from build123d import *

# Parameters (mm, degrees)
SKETCH1_R           = 1.6
BOSS_EXTRUDE1_DEPTH = 8
CHAMFER1_SIZE       = 1
SKETCH2_R           = 1.6
BOSS_EXTRUDE3_DEPTH = 8
FILLET1_R           = 10
CHAMFER2_SIZE       = 1


with BuildPart() as part:
    # Sketch1 → Boss-Extrude1 (new body)
    with BuildSketch(Plane.XY):
        with BuildLine():
            Line((-0.5, 3), (30.5, 3))
            ThreePointArc((30.5, 3), (32.267766953, 2.267766953), (33, 0.5))
            Line((33, 0.5), (33, -0.5))
            ThreePointArc((33, -0.5), (32.267766953, -2.267766953), (30.5, -3))
            Line((30.5, -3), (-0.5, -3))
            ThreePointArc((-0.5, -3), (-2.267766953, -2.267766953), (-3, -0.5))
            Line((-3, -0.5), (-3, 0.5))
            ThreePointArc((-3, 0.5), (-2.267766953, 2.267766953), (-0.5, 3))
        make_face()
        Circle(SKETCH1_R, mode=Mode.SUBTRACT)
        with Locations((7.5, 0)):
            Circle(SKETCH1_R, mode=Mode.SUBTRACT)
        with Locations((15, 0)):
            Circle(SKETCH1_R, mode=Mode.SUBTRACT)
        with Locations((22.5, 0)):
            Circle(SKETCH1_R, mode=Mode.SUBTRACT)
        with Locations((30, 0)):
            Circle(SKETCH1_R, mode=Mode.SUBTRACT)
    extrude(amount=BOSS_EXTRUDE1_DEPTH)

    # Chamfer1
    chamfer1_edges = [part.edges().sort_by_distance(p)[0] for p in [
        (-1.6, 0, 0),
        (-1.6, 0, 8),
        (5.9, 0, 0),
        (5.9, 0, 8),
        (13.4, 0, 0),
        (13.4, 0, 8),
        (20.9, 0, 0),
        (20.9, 0, 8),
        (28.4, 0, 0),
        (28.4, 0, 8),
    ]]
    chamfer(chamfer1_edges, length=CHAMFER1_SIZE)

    # Sketch2 → Boss-Extrude3 (add)
    with BuildSketch(Plane.XY.offset(8)):
        with BuildLine():
            ThreePointArc((-3, 0.5), (-2.809698831, 1.456708581), (-2.267766953, 2.267766953))
            Line((-2.267766953, 2.267766953), (-18.529200529, -13.993666623))
            ThreePointArc((-18.529200529, -13.993666623), (-19.261433576, -15.761433576), (-18.529200529, -17.529200529))
            Line((-18.529200529, -17.529200529), (-17.822093748, -18.23630731))
            ThreePointArc((-17.822093748, -18.23630731), (-16.054326795, -18.968540357), (-14.286559842, -18.23630731))
            Line((-14.286559842, -18.23630731), (0.949747468, -3))
            Line((0.949747468, -3), (-0.5, -3))
            ThreePointArc((-0.5, -3), (-2.267766953, -2.267766953), (-3, -0.5))
            Line((-3, -0.5), (-3, 0.5))
        make_face()
        with Locations((-16.054326795, -15.761433576)):
            Circle(SKETCH2_R, mode=Mode.SUBTRACT)
        with Locations((-10.751025936, -10.458132717)):
            Circle(SKETCH2_R, mode=Mode.SUBTRACT)
        with Locations((-5.447725077, -5.154831858)):
            Circle(SKETCH2_R, mode=Mode.SUBTRACT)
    extrude(amount=-BOSS_EXTRUDE3_DEPTH)

    # Fillet1
    fillet1_edges = [part.edges().sort_by_distance(p)[0] for p in [
        (0.949747468, -3, 4),
    ]]
    fillet(fillet1_edges, radius=FILLET1_R)

    # Chamfer2
    chamfer2_edges = [part.edges().sort_by_distance(p)[0] for p in [
        (-17.654326795, -15.761433576, 8),
        (-12.351025936, -10.458132717, 8),
        (-7.047725077, -5.154831858, 8),
        (-7.047725077, -5.154831858, 0),
        (-12.351025936, -10.458132717, 0),
        (-17.654326795, -15.761433576, 0),
    ]]
    chamfer(chamfer2_edges, length=CHAMFER2_SIZE)


solid = part.part
Model file for the job. Use its own axes, mm. Coordinates: 2 decimals unless noted, no trailing zeros. Loops run counter-clockwise (first coordinate to the right, second up) from the corner with the lowest first, then second, coordinate; pieces in that order, holes last. Notation, with made-up numbers: (-25.5, -17) -> (-6.5, -17) arc R9 cw to (-6.5, -13) -> close; hole circle Ø4 at (29, -34.5). An arc over 180 degrees is marked (long way). Use one line per item in the form item = value. Start each with the question number.
(1) Cut at A-A on x = 30. Give the cut face in (y, z).
(2) Flat gauge pins, fed straight in: pin 1 (1 mm diameter, centred on x = -6.5, z = 2, fed in from +Y); pin 2 (1 mm diameter, centred on y = -13, z = 1.5, fed in from +X); pin 3 (5 mm diameter, centred on x = 22.5, y = 0, fed in from -Z). Where does each tip first touch, or does it go through?
(3) Cut at B-B on z = 4. Give the number of separate pieces and of enclosed holes in the cut face, and give its area (3 significant figures).
(4) Pull direction Y, two halves, no side cores. Call faces 1 (the cylindrical face through (32.248, 2.287, 3.944)), 2 (the flat face through (33, 0, 4)), 3 (the cylindrical face through (13.4, 0.07, 3.96)): pulls with the +Y half, pulls with the -Y half, needs draft (parallel to the pull), parting line crosses it, or undercut.
(5) Probe probe 1 along Y at (x, z) = (30, 3.8); probe 2 along X at (y, z) = (-1.25, 4.5); probe 3 along Y at (x, z) = (5, 6.5). List the from-to ranges inside material, lowest first. Write a range as from..to.
Values:
q1.outline = (-3, 0) -> (-2.6, 0) -> (-1.6, 1) -> (-1.6, 7) -> (-2.6, 8) -> (-3, 8) -> close; (1.6, 1) -> (2.6, 0) -> (3, 0) -> (3, 8) -> (2.6, 8) -> (1.6, 7) -> close
q2.pin_1 = -1.46
q2.pin_2 = -8.55
q2.pin_3 = 0.1
q3.separate_pieces = 1
q3.enclosed_holes = 8
q3.area = 284 mm2
q4.face_1 = pulls with the +Y half
q4.face_2 = needs draft
q4.face_3 = undercut
q5.probe_1 = -3..-1.6, 1.6..3
q5.probe_2 = -5.79..-1, 1..6.5, 8.5..14, 16..21.5, 23.5..29, 31..32.88
q5.probe_3 = -3..3
